Verification items for the finished model (mm, model axes). Face numbers are marked on the shaded views. A direction names the side the tool comes from. Give positions to 0.01 mm unless a question says otherwise; leave off trailing zeros. Write each loop counter-clockwise with the first axis right and the second up, starting at its lowest first coordinate (ties: lowest second). Pieces come first, ordered by that corner, then holes. Notation, with made-up numbers: (49, 81) - (89, 81) arc R22 cw to (89, 116) - close; hole circle Ø4 at (14, 79.25). An arc over 180 degrees is marked (long way). Put each result on its own line as item: value.
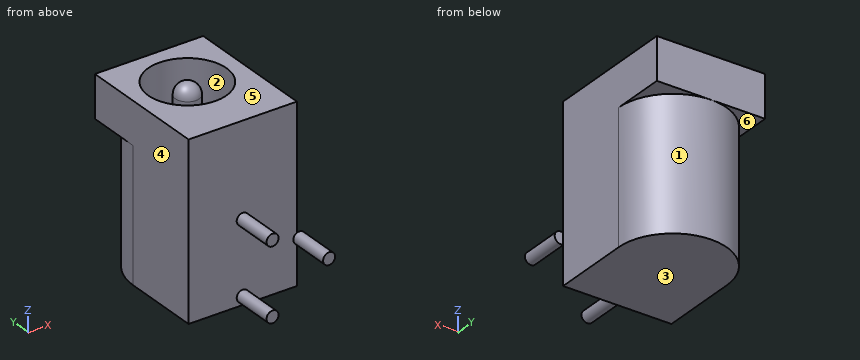
from build123d import *

# Parameters (mm, degrees)
BOSS_EXTRUDE1_DEPTH = 14.4
SKETCH3_W           = 9
SKETCH3_H           = 4.5
BOSS_EXTRUDE2_DEPTH = 3.5
SKETCH2_R           = 3.25
SKETCH2_R_2         = 1
CUT_EXTRUDE1_DEPTH  = 10
FILLET1_R           = 1
SKETCH4_R           = 0.5
BOSS_EXTRUDE3_DEPTH = 3.5


with BuildPart() as part:
    # Sketch1 → Boss-Extrude1 (new body)
    with BuildSketch(Plane.XY):
        with BuildLine():
            Line((4.5, 0), (-4.5, 0))
            Line((-4.5, 0), (-4.5, 6.5))
            ThreePointArc((-4.5, 6.5), (0, 11), (4.5, 6.5))
            Line((4.5, 6.5), (4.5, 0))
        make_face()
    extrude(amount=-BOSS_EXTRUDE1_DEPTH)

    # Sketch3 → Boss-Extrude2 (add)
    with BuildSketch(Plane.XY):
        with Locations((0, 8.75)):
            Rectangle(SKETCH3_W, SKETCH3_H)
    extrude(amount=-BOSS_EXTRUDE2_DEPTH)

    # Sketch2 → Cut-Extrude1 (cut)
    with BuildSketch(Plane.XY):
        with Locations((0, 6.5)):
            Circle(SKETCH2_R)
        with Locations((0, 6.5)):
            Circle(SKETCH2_R_2, mode=Mode.SUBTRACT)
    extrude(amount=-CUT_EXTRUDE1_DEPTH, mode=Mode.SUBTRACT)

    # Fillet1
    fillet1_edges = [part.edges().sort_by_distance(p)[0] for p in [
        (-1, 6.5, 0),
    ]]
    fillet(fillet1_edges, radius=FILLET1_R)

    # Sketch4 → Boss-Extrude3 (add)
    with BuildSketch(Plane.XZ):
        with Locations((0, -13.7)):
            Circle(SKETCH4_R)
        with Locations((0, -7.7)):
            Circle(SKETCH4_R)
        with Locations((4.7, -10.7)):
            Circle(SKETCH4_R)
    extrude(amount=BOSS_EXTRUDE3_DEPTH)


solid = part.part
Q1. Set-up check for the marked faces 5 and 6: record each of +Z, -Z, +X, -X, +Y, -Y from which the full face is reachable in a straight line by a thin tool's end or side.
Answers follow:
face 5: +Z, +X, -X, +Y, -Y
face 6: -Z, -X, +Y
Q2. Release check for a two-part mould opening along X. For the marked faces 1, 2, 3 and 4 record: released by +X, released by -X, zero draft, split by the parting line, or undercut.
Answers follow:
face 1: split by the parting line
face 2: undercut
face 3: zero draft
face 4: released by -X
Q3. Section check D-D, the plane x = -2. Record the cut outline in (y, z), plus the area to 3 significant figures.
Answers follow:
outline: (0, -14.4) - (10.53, -14.4) - (10.53, -3.5) - (11, -3.5) - (11, 0) - (9.06, 0) - (9.06, -10) - (3.94, -10) - (3.94, 0) - (0, 0) - close
area: 102 mm2
Q4. Go/stop test with flat-tipped pins: pin 1 Ø1.5 at (x, z) = (1.5, -9) entering from +Y; pin 2 Ø0.8 at (x, z) = (5, -10.5) entering from +Y; pin 3 Ø3 at (x, z) = (-3, -12.5) entering from +Y. Record where each tip stops, or that it passes through.
Answers follow:
pin 1: stops at y = 10.94
pin 2: stops at y = 0
pin 3: stops at y = 10.74
Q5. Section check A-A, the plane z = -9.5. Record the cut outline in (x, y).
Answers follow:
outline: (-4.5, 0) - (4.5, 0) - (4.5, 6.5) arc R4.5 ccw to (-4.5, 6.5) - close; circle Ø2 at (0, 6.5); hole circle Ø6.5 at (0, 6.5)
Q6. Section check B-B, the plane y = -0.75. Record the cut outline in (x, z).
Answers follow:
outline: circle Ø1 at (0, -13.7); circle Ø1 at (0, -7.7); circle Ø1 at (4.7, -10.7)
Q7. Scan lines: line 1 along Y through (x, z) = (0, -3.25); line 2 along Y through (x, z) = (-0.75, -9.25); line 3 along X through (y, z) = (6.25, -6.5). Record each from-to range of solid material in increasing order.
Answers follow:
line 1: y = 0 to 3.25, 5.5 to 7.5, 9.75 to 11
line 2: y = 0 to 3.34, 5.84 to 7.16, 9.66 to 10.94
line 3: x = -4.5 to -3.24, -0.97 to 0.97, 3.24 to 4.5
Q8. Section check C-C, the plane z = -13.7. Record the cut outline in (x, y).
Answers follow:
outline: (-4.5, 0) - (-0.5, 0) - (-0.5, -3.5) - (0.5, -3.5) - (0.5, 0) - (4.5, 0) - (4.5, 6.5) arc R4.5 ccw to (-4.5, 6.5) - close
